Design review of the part built by this model. Coordinates are the model's own, in mm. A direction names the side the tool comes from. Coordinates: 2 decimals unless noted, no trailing zeros. Loops run counter-clockwise (first coordinate to the right, second up) from the corner with the lowest first, then second, coordinate; pieces in that order, holes last. Notation, with made-up numbers: (40, 13.25) -> (73, 13.25) arc R24 cw to (73, 44.25) -> close; hole circle Ø6 at (67.25, -0.5). An arc over 180 degrees is marked (long way). Answer as a JSON object with one key per item and string values.
Autodesk Inventor part; units mm, degrees
ref_plane "Work Plane1" through (55, 0, 10) normal (0, 0, 1) x (1, 0, 0)
ref_plane "YZ Plane" through (0, 0, 0) normal (1, 0, 0) x (0, 1, 0)
ref_plane "XZ Plane" through (0, 0, 0) normal (0, 1, 0) x (-1, 0, 0)
sketch "Sketch1" plane through (0, 0, 0) normal (0, 1, 0) x (-1, 0, 0)
  line L0 (0, 0) -> (-55, 0)
  line L1 (-55, 0) -> (-55, 20)
  line L2 (-55, 20) -> (0, 20)
  line L3 (0, 20) -> (0, 0)
  dimension "d0" = 55
  dimension "d1" = 20
extrude "Extrusion1" add sketch "Sketch1" along normal blind 3
sketch "Sketch2" plane through (0, 3, 0) normal (0, 1, 0) x (1, 0, 0)
  line L0 (0, -20) -> (55, -20)
  line L1 (55, -20) -> (55, 0)
  line L2 (44.5, -20) -> (39.5, -20)
  line L3 (39.5, -20) -> (39.5, -17)
  line L4 (39.5, -17) -> (44.5, -17)
  line L5 (44.5, -17) -> (44.5, -20)
  line L6 (30, -20) -> (25, -20)
  line L7 (25, -20) -> (25, -17)
  line L8 (25, -17) -> (30, -17)
  line L9 (30, -17) -> (30, -20)
  line L10 (15.5, -20) -> (10.5, -20)
  line L11 (10.5, -20) -> (10.5, -17)
  line L12 (10.5, -17) -> (15.5, -17)
  line L13 (15.5, -17) -> (15.5, -20)
  point P0 (0, 0)
  dimension "d5" = 3
  dimension "d7" = 3
  dimension "d9" = 3
  dimension "d13" = 55
  dimension "d16" = 34
  dimension "d17" = 9.5
  dimension "d18" = 9.5
  dimension "d19" = 5
  dimension "d20" = 5
  dimension "d21" = 10.5
extrude "Extrusion2" cut sketch "Sketch2" against normal blind 3
ref_plane "Work Plane1" through (55, 0, 10) normal (0, 0, 1) x (1, 0, 0)
mirror "Mirror1" about plane through (55, 0, 10) normal (0, 0, 1) of "Extrusion2"
equation "\"d18\" = d17"
equation "\"d20\" = d19"
equation "\"d21\" = -d17 + 0.5 * d13 - 1.5 * d19"
properties part number "unionpress" material "Glass"
1) Wall thickness on probe 1 along X at (y, z) = (1.3, 2.25); probe 2 along Z at (x, y) = (13.5, 1.65): over which ranges is each line inside the solid? List them lowest first.
Completed:
{"probe 1": "0 to 10.5, 15.5 to 25, 30 to 39.5, 44.5 to 55", "probe 2": "3 to 17"}
2) Add section A-A, the plane y = 1. Give the boundary of the cut face in (x, z).
Completed:
{"outline": "(0, 0) -> (10.5, 0) -> (10.5, 3) -> (15.5, 3) -> (15.5, 0) -> (25, 0) -> (25, 3) -> (30, 3) -> (30, 0) -> (39.5, 0) -> (39.5, 3) -> (44.5, 3) -> (44.5, 0) -> (55, 0) -> (55, 20) -> (44.5, 20) -> (44.5, 17) -> (39.5, 17) -> (39.5, 20) -> (30, 20) -> (30, 17) -> (25, 17) -> (25, 20) -> (15.5, 20) -> (15.5, 17) -> (10.5, 17) -> (10.5, 20) -> (0, 20) -> close"}
3) Add section B-B, the plane x = 40. Give the boundary of the cut face in (y, z), and give its area (3 significant figures).
Completed:
{"outline": "(0, 3) -> (3, 3) -> (3, 17) -> (0, 17) -> close", "area": "42.0 mm²"}
4) For faces 4 (the flat face through (28, 0, 10)), 5 (the flat face through (30, 2, 18)), 6 (the flat face through (42, 2, 3)), list the 3-axis set-ups (+Z, -Z, +X, -X, +Y, -Y) from which the entire face can be reached by the end or side of a thin tool; tool diameter is ignored.
Completed:
{"face 4": "+Z, -Z, +X, -X, -Y", "face 5": "+Z, +Y, -Y", "face 6": "-Z, +Y, -Y"}
5) Clearance check with flat-ended pins moving along their axes: pin 1 Ø0.9 at (y, z) = (2, 18.5) entering from -X; pin 2 Ø0.9 at (x, y) = (13, 1) entering from -Z; pin 3 Ø0.9 at (x, y) = (12, 1) entering from +Z. State where each tip first meets the part, or that it passes through.
Completed:
{"pin 1": "x = 0", "pin 2": "z = 3", "pin 3": "z = 17"}
6) The part is to be moulded in two halves that separate along X. For faces 1 (the flat face through (50, 1, 0)), 2 (the flat face through (13, 2, 17)), 3 (the flat face through (55, 1, 10)), say which applies: pulls with the +X half, pulls with the -X half, needs draft (parallel to the pull), parting line crosses it, or undercut.
Completed:
{"face 1": "needs draft", "face 2": "undercut", "face 3": "pulls with the +X half"}
